Read the model definition and answer for the solid it produces. Units are mm, in the model's axes. Give positions to 0.01 mm unless a question says otherwise; leave off trailing zeros. Order: outer loops, then holes, each group sorted by start corner. A loop starts at its lowest first (then second) coordinate and runs counter-clockwise, first axis right, second up. Notation, with made-up numbers: (19, 4.25) - (24, 4.25) arc R9 cw to (24, 9.25) - close; hole circle Ø1 at (-19.5, -25.5). An arc over 180 degrees is marked (long way). Write each question's results on one line, items separated by ' | '. Start each with the question number.
Q1. Find section A-A on z = 30.5. Give the vertices of the cut face in (x, y).
Q2. Find the intervals of material crossed by line 1 along Y through (x, z) = (60, 5); line 2 along Y through (x, z) = (-60, 11.5); line 3 along X through (y, z) = (-12, 128), in increasing order. Write a range as from..to.
Q3. Flat-ended cylindrical pins translate along their axes: P1, Ø16, axis at x = 61.5, y = -139, coming from the +Z side; P2, Ø25, axis at x = -67, y = -141, coming from the +Z side; P3, Ø2, axis at x = 59.5, z = 254, coming from the -Y side; P4, Ø12.5, axis at x = -72, z = 200, coming from the -Y side. Find the tip coordinate at first contact, or state that the pin passes through.
Q4. Find section B-B on y = -260. Give the vertices of the cut face in (x, z).
Q5. Find section C-C on z = 128. Give the vertices of the cut face in (x, y).
Q6. Find section D-D on y = -94.5. Give the vertices of the cut face in (x, z).
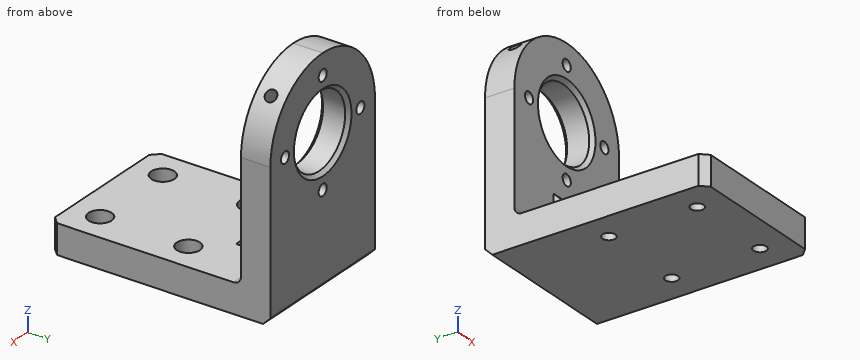
from build123d import *

# Parameters (mm, degrees)
F0_R            = 7.5770017359
F0_R_2          = 50
F1_DEPTH        = 40
F2_D            = 15.5
F2_DEPTH        = 40
F2_TIP          = 4.6566697975
F3_SIZE         = 5
F9_D            = 15.5
F9_DEPTH        = 40
F9_START        = 0.3007649
F9_TIP          = 4.6566697975
F11_D           = 15.5
F11_DEPTH       = 40
F11_START       = 0.3007649
F11_TIP         = 4.6566697975
F12_W           = 300
F12_H           = 40
F13_DEPTH       = 100
F15_R           = 10
F16_DEPTH       = 25
F17_SIZE        = 10
F19_D           = 17.5
F19_CBORE_D     = 31.5
F19_CBORE_DEPTH = 20


with BuildPart() as f1:
    # F0 (on Front) → F1 (new body)
    with BuildSketch(Plane.XZ):
        with BuildLine():
            Line((-100, 200), (-100, 0))
            Line((-100, 0), (100, 0))
            Line((100, 0), (100, 200))
            ThreePointArc((100, 200), (70.7106781187, 270.7106781187), (0, 300))
            ThreePointArc((0, 300), (-70.7106781187, 270.7106781187), (-100, 200))
        make_face()
        with Locations((0, 128)):
            Circle(F0_R, mode=Mode.SUBTRACT)
        with Locations((-72, 200)):
            Circle(F0_R, mode=Mode.SUBTRACT)
        with Locations((0, 200)):
            Circle(F0_R_2, mode=Mode.SUBTRACT)
        with Locations((72, 200)):
            Circle(F0_R, mode=Mode.SUBTRACT)
        with Locations((0, 272)):
            Circle(F0_R, mode=Mode.SUBTRACT)
        with Locations((72, 200)):
            Circle(F0_R)
        with Locations((0, 128)):
            Circle(F0_R)
        with Locations((-72, 200)):
            Circle(F0_R)
        with Locations((0, 272)):
            Circle(F0_R)
    extrude(amount=F1_DEPTH)

    # F2
    with Locations(Plane(origin=(0, 0, 0), x_dir=(1, 0, 0), z_dir=(0, 1, 0))):
        with Locations((0, -272), (72, -200), (0, -128), (-72, -200)):
            Hole(F2_D / 2, depth=F2_DEPTH)
            with Locations((0, 0, -(F2_DEPTH + F2_TIP / 2))):  # 118° drill point
                Cone(0, F2_D / 2, F2_TIP, mode=Mode.SUBTRACT)

    # F3
    f3_edges = [f1.edges().sort_by_distance(p)[0] for p in [
        (-50, 0, 200),
        (-50, -40, 200),
    ]]
    chamfer(f3_edges, length=F3_SIZE)

    # F9
    # its depths count from where the whole tool has entered the part; down to there all is cleared
    with Locations(Plane(origin=(170.7106781187, 0, 170.7106781187), x_dir=(0.7071067812, 0, -0.7071067812), z_dir=(0.7071067812, 0, 0.7071067812)).offset(-F9_START)):
        with Locations((-141.4213562373, -20)):
            Hole(F9_D / 2, depth=F9_DEPTH)
            with Locations((0, 0, -(F9_DEPTH + F9_TIP / 2))):  # 118° drill point
                Cone(0, F9_D / 2, F9_TIP, mode=Mode.SUBTRACT)

    # F11
    # its depths count from where the whole tool has entered the part; down to there all is cleared
    with Locations(Plane(origin=(-170.7106781187, 0, 170.7106781187), x_dir=(0, -1, 0), z_dir=(-0.7071067812, 0, 0.7071067812)).offset(-F11_START)):
        with Locations((20, 141.4213562373)):
            Hole(F11_D / 2, depth=F11_DEPTH)
            with Locations((0, 0, -(F11_DEPTH + F11_TIP / 2))):  # 118° drill point
                Cone(0, F11_D / 2, F11_TIP, mode=Mode.SUBTRACT)

    # F12 (on Right) → F13 (join, symmetric)
    with BuildSketch(Plane.YZ):
        with Locations((-150, 20)):
            Rectangle(F12_W, F12_H)
    extrude(amount=F13_DEPTH, both=True)

    # F15
    f15_edges = [f1.edges().sort_by_distance(p)[0] for p in [
        (0, -40, 40),
    ]]
    fillet(f15_edges, radius=F15_R)

    # F14 (on Right) → F16 (join, symmetric)
    with BuildSketch(Plane.YZ):
        Polygon((-40, 40), (-40, 100), (-100, 40), align=None)
    extrude(amount=F16_DEPTH, both=True)

    # F17
    f17_edges = [f1.edges().sort_by_distance(p)[0] for p in [
        (100, -300, 20),
        (-100, -300, 20),
        (0, 0, 0),
    ]]
    chamfer(f17_edges, length=F17_SIZE)

    # F19 (through all)
    with Locations(Plane.XY.offset(40)):
        with Locations((-60, -140), (60, -140), (60, -260), (-60, -260)):
            CounterBoreHole(F19_D / 2, F19_CBORE_D / 2, F19_CBORE_DEPTH)


solid = f1.part
Working result:
1) outline: (-100, -290) - (-90, -300) - (90, -300) - (100, -290) - (100, 0) - (-100, 0) - close; hole circle Ø31.5 at (-60, -260); hole circle Ø31.5 at (-60, -140); hole circle Ø31.5 at (60, -260); hole circle Ø31.5 at (60, -140)
2) line 1: -300..-268.75, -251.25..-148.75, -131.25..-5 | line 2: -300..-268.75, -251.25..-148.75, -131.25..0 | line 3: -100..-7.75, 7.75..100
3) P1: z = 20 | P2: z = 40 | P3: y = -40 | P4: through
4) outline: (-100, 0) - (-68.75, 0) - (-68.75, 20) - (-75.75, 20) - (-75.75, 40) - (-100, 40) - close; (-51.25, 0) - (51.25, 0) - (51.25, 20) - (44.25, 20) - (44.25, 40) - (-44.25, 40) - (-44.25, 20) - (-51.25, 20) - close; (68.75, 0) - (100, 0) - (100, 40) - (75.75, 40) - (75.75, 20) - (68.75, 20) - close
5) outline: (-100, -40) - (-7.75, -40) - (-7.75, 0) - (-100, 0) - close; (7.75, -40) - (100, -40) - (100, 0) - (7.75, 0) - close
6) outline: (-100, 0) - (100, 0) - (100, 40) - (25, 40) - (25, 45.5) - (-25, 45.5) - (-25, 40) - (-100, 40) - close
